Geometry: final body of the model. Coordinates: model frame, mm. A direction names the side the tool comes from. Give positions to 0.01 mm unless a question says otherwise; leave off trailing zeros. Write each loop counter-clockwise with the first axis right and the second up, starting at its lowest first coordinate (ties: lowest second). Pieces come first, ordered by that corner, then holes. Notation, with made-up numbers: M -3.75,-21 L 38.25,-21 A23 cw 38.25,3 Z; hole C 13.5,16.25 d6. An arc over 180 degrees is marked long. Answer as a JSON object with one key per item and string values.
from build123d import *
from build123d.topology import SkipClean

# Parameters (mm, degrees)
ESQUISSE1_R           = 15
ESQUISSE1_R_2         = 5
ESQUISSE1_R_3         = 2
EXTRUSION1_DEPTH      = 6.5
ESQUISSE2_R           = 9
ESQUISSE2_R_2         = 1.5
EXTRUSION2_DEPTH      = 30
ESQUISSE3_R           = 15
EXTRUSION3_DEPTH      = 27
EXTRUSION4_DEPTH      = 104.717163478
EXTRUSION4_DEPTH_BACK = 104.717163478
EXTRUSION5_DEPTH      = 104.717163478
ESQUISSE6_W           = 10
ESQUISSE6_H           = 15
EXTRUSION6_DEPTH      = 59.883359279


with BuildPart() as part:
    # Esquisse1 → Extrusion1 (new body)
    with BuildSketch(Plane.XY):
        with BuildLine():
            Line((20, -20), (20, -75))
            ThreePointArc((20, -75), (0, -95), (-20, -75))
            Line((-20, -75), (-20, -20))
            ThreePointArc((-20, -20), (0, 0), (20, -20))
        make_face()
        with Locations(Location((0, -75, 0), (0, 0, 180))):
            Circle(ESQUISSE1_R, mode=Mode.SUBTRACT)
        with Locations(Location((0, -20, 0), (0, 0, 180))):
            Circle(ESQUISSE1_R_2, mode=Mode.SUBTRACT)
        with Locations(Location((-14, -20, 0), (0, 0, 180))):
            Circle(ESQUISSE1_R_3, mode=Mode.SUBTRACT)
        with Locations(Location((-9.899494937, -10.100505063, 0), (0, 0, 180))):
            Circle(ESQUISSE1_R_3, mode=Mode.SUBTRACT)
        with Locations(Location((0, -6, 0), (0, 0, 180))):
            Circle(ESQUISSE1_R_3, mode=Mode.SUBTRACT)
        with Locations(Location((9.899494937, -10.100505063, 0), (0, 0, 180))):
            Circle(ESQUISSE1_R_3, mode=Mode.SUBTRACT)
        with Locations(Location((14, -20, 0), (0, 0, 180))):
            Circle(ESQUISSE1_R_3, mode=Mode.SUBTRACT)
        with Locations(Location((9.899494937, -29.899494937, 0), (0, 0, 180))):
            Circle(ESQUISSE1_R_3, mode=Mode.SUBTRACT)
        with Locations(Location((0, -34, 0), (0, 0, 180))):
            Circle(ESQUISSE1_R_3, mode=Mode.SUBTRACT)
        with Locations(Location((-9.899494937, -29.899494937, 0), (0, 0, 180))):
            Circle(ESQUISSE1_R_3, mode=Mode.SUBTRACT)
    extrude(amount=EXTRUSION1_DEPTH)

    # Esquisse2 → Extrusion2 (add)
    with SkipClean():  # the faces are left unmerged after this step: merging them gives an invalid solid
        with BuildSketch(Plane.XY.offset(6.5)):
            with BuildLine():
                Line((12, -59), (-12, -59))
                ThreePointArc((-12, -59), (0, -95), (12, -59))
            make_face()
            with Locations((0, -75)):
                Circle(ESQUISSE2_R, mode=Mode.SUBTRACT)
            with Locations((0, -62)):
                Circle(ESQUISSE2_R_2, mode=Mode.SUBTRACT)
            with Locations((0, -88)):
                Circle(ESQUISSE2_R_2, mode=Mode.SUBTRACT)
            with Locations((-13, -75)):
                Circle(ESQUISSE2_R_2, mode=Mode.SUBTRACT)
            with Locations((13, -75)):
                Circle(ESQUISSE2_R_2, mode=Mode.SUBTRACT)
        extrude(amount=EXTRUSION2_DEPTH)

    # Esquisse3 → Extrusion3 (cut)
    with SkipClean():  # the faces are left unmerged after this step: merging them gives an invalid solid
        with BuildSketch(Plane(origin=(0, 0, 6.5), x_dir=(-1, 0, 0), z_dir=(0, 0, -1))):
            with Locations((0, -75)):
                Circle(ESQUISSE3_R)
        extrude(amount=-EXTRUSION3_DEPTH, mode=Mode.SUBTRACT)

    # Esquisse4 → Extrusion4 (cut, two sides: drawn at the far end of the back side and taken through both)
    with SkipClean():  # the faces are left unmerged after this step: merging them gives an invalid solid
        with BuildSketch(Plane(origin=(0, 0, 0), x_dir=(0, 0, -1), z_dir=(1, 0, 0)).offset(-EXTRUSION4_DEPTH_BACK)):
            Polygon((-36.5, -95), (-30, -95), (-36.5, -90), align=None)
        extrude(amount=EXTRUSION4_DEPTH + EXTRUSION4_DEPTH_BACK, mode=Mode.SUBTRACT)

    # Esquisse5 → Extrusion5 (cut, through all)
    with BuildSketch(Plane.XY.offset(36.5)):
        with BuildLine():
            Line((20, -55), (-20, -55))
            Line((-20, -55), (-20, -75))
            ThreePointArc((-20, -75), (0, -95), (20, -75))
            Line((20, -75), (20, -55))
        make_face()
    extrude(amount=-EXTRUSION5_DEPTH, mode=Mode.SUBTRACT)

    # Esquisse6 → Extrusion6 (cut, through all)
    with BuildSketch(Plane.XY.offset(6.5)):
        with Locations((-15, -47.5)):
            Rectangle(ESQUISSE6_W, ESQUISSE6_H)
        with Locations((15, -47.5)):
            Rectangle(ESQUISSE6_W, ESQUISSE6_H)
    extrude(amount=-EXTRUSION6_DEPTH, mode=Mode.SUBTRACT)


solid = part.part
1) Cut plane D-D on z = 5.25. Give the number of separate pieces and of enclosed holes in the cut face, and give its area (3 significant figures).
Geometry check:
{"separate pieces": "1", "enclosed holes": "9", "area": "1,550 mm2"}
2) Cut plane B-B on y = -23. Return loops of the section in (x, z).
Geometry check:
{"outline": "M -20,0 L -4,0 L -4,6.5 L -20,6.5 Z; M 4,0 L 20,0 L 20,6.5 L 4,6.5 Z"}
3) Set-up query: faces 5 (the flat face through (-15, -40, 3)), 6 (the flat face through (15, -40, 3)), 7 (the cylindrical face through (0, -8, 3)). Return all of +Z, -Z, +X, -X, +Y, -Y with unobstructed straight access to the full face (end or side cutting, diameter ignored); none if empty.
Geometry check:
{"face 5": "+Z, -Z, -X, -Y", "face 6": "+Z, -Z, +X, -Y", "face 7": "+Z, -Z"}
4) Line query: line 1 (Y direction, x = 0, z = 4.75); line 2 (X direction, y = -34, z = 3); line 3 (X direction, y = -19, z = 6). Output: solid intervals per line, ascending. Write a range as from..to.
Geometry check:
{"line 1": "y = -55..-36, -32..-25, -15..-8, -4..0", "line 2": "x = -20..-2, 2..20", "line 3": "x = -19.97..-15.73, -12.27..-4.9, 4.9..12.27, 15.73..19.97"}
5) Cut plane C-C on x = -14. Return loops of the section in (y, z), and give its area (3 significant figures).
Geometry check:
{"outline": "M -40,0 L -22,0 L -22,6.5 L -40,6.5 Z; M -18,0 L -5.72,0 L -5.72,6.5 L -18,6.5 Z", "area": "197 mm2"}
6) Contact query for flat-ended pins moving along their axis: P1, Ø2, axis at y = -47, z = 4, coming from the -X side; P2, Ø2, axis at x = 14, z = 2, coming from the -Y side; P3, Ø3.5, axis at x = 14, y = -20, coming from the -Z side. Output: stop coordinate, or through.
Geometry check:
{"P1": "stops at x = -10", "P2": "stops at y = -40", "P3": "passes through"}
7) Cut plane A-A on x = 0. Return loops of the section in (y, z).
Geometry check:
{"outline": "M -55,0 L -36,0 L -36,6.5 L -55,6.5 Z; M -32,0 L -25,0 L -25,6.5 L -32,6.5 Z; M -15,0 L -8,0 L -8,6.5 L -15,6.5 Z; M -4,0 L 0,0 L 0,6.5 L -4,6.5 Z"}
8) Pull-direction query (X, two-part tool) for faces 1 (the flat face through (-20, -30, 3)), 2 (the flat face through (0, -55, 3)), 3 (the cylindrical face through (-14, -22, 3)), 4 (the cylindrical face through (0, 0, 3)); classes: pulls with the +X half, pulls with the -X half, needs draft (parallel to the pull), parting line crosses it, or undercut.
Geometry check:
{"face 1": "pulls with the -X half", "face 2": "needs draft", "face 3": "undercut", "face 4": "parting line crosses it"}
